```python
from build123d import *

# Parameters (mm, degrees)
SKETCH1_R           = 1.75
BOSS_EXTRUDE1_DEPTH = 12
SKETCH3_R           = 1.6
CUT_EXTRUDE1_DEPTH  = 3.5
BOSS_EXTRUDE2_DEPTH = 12


with BuildPart() as part:
    # Sketch1 → Boss-Extrude1 (new body)
    with BuildSketch(Plane(origin=(0, 0, 0), x_dir=(1, 0, 0), z_dir=(0, 1, 0))):
        Polygon((-1.649648438, 29.291322314), (-1.649648438, -3.708677686), (3.350351562, -3.708677686), (3.350351562, 31.791322314), (-26.649648438, 31.791322314), (-26.649648438, 29.291322314), align=None)
        with Locations((0.850351562, -1.208677686)):
            Circle(SKETCH1_R, mode=Mode.SUBTRACT)
    extrude(amount=BOSS_EXTRUDE1_DEPTH)

    # Sketch3 → Cut-Extrude1 (cut, through all)
    with BuildSketch(Plane.XY.offset(-29.291322314)):
        with Locations((-21.379789069, 2.5)):
            Circle(SKETCH3_R)
        with Locations((-21.379789069, 9.5)):
            Circle(SKETCH3_R)
    extrude(amount=-CUT_EXTRUDE1_DEPTH, mode=Mode.SUBTRACT)

    # Sketch4 → Boss-Extrude2 (add, through all)
    with BuildSketch(Plane(origin=(0, 0, 0), x_dir=(1, 0, 0), z_dir=(0, 1, 0))):
        Polygon((-1.649648438, 4.291322314), (-4.149648438, 4.291322314), (-4.149648438, -6.208677686), (5.850351562, -6.208677686), (5.850351562, 3.519074646), (3.350351562, 3.519074646), (3.350351562, -3.708677686), (-1.649648438, -3.708677686), align=None)
    extrude(amount=BOSS_EXTRUDE2_DEPTH)


solid = part.part
```
Design review of the part built by this model. Coordinates are the model's own, in mm. A direction names the side the tool comes from. Coordinates: 2 decimals unless noted, no trailing zeros. Order: outer loops, then holes, each group sorted by start corner. A loop starts at its lowest first (then second) coordinate and runs counter-clockwise, first axis right, second up.
1) Take a section at C-C, the plane z = -21.5. Give the boundary of the cut face in (x, y), and give its area (3 significant figures).
2) Take a section at A-A, the plane y = 2. Give the boundary of the cut face in (x, z), and give its area (3 significant figures).
3) Take a section at B-B, the plane y = 7. Give the boundary of the cut face in (x, z), and give its area (3 significant figures).
4) For faces 5 (the flat face through (-4.15, 6, 1)), 6 (the flat face through (5, 6, -3.519)), 7 (the flat face through (-3, 6, -4.291)), list the 3-axis set-ups (+Z, -Z, +X, -X, +Y, -Y) from which the entire face can be reached by the end or side of a thin tool; tool diameter is ignored.
5) Take a section at D-D, the plane x = -13. Give the boundary of the cut face in (y, z).
6) Mouldability with a two-part tool opening along Z and no side actions: class faces 1 (the flat face through (-1.65, 6, -17)), 2 (the flat face through (1, 6, 6.209)), 3 (the cylindrical face through (-0.54, 5.92, 2.27)), 4 (the flat face through (-1, 0, -16)) as +Z half, -Z half, draft (parallel to the pull), parting line (faces both ways), or undercut.
7) Wall thickness on line 1 along Z through (x, y) = (-3.5, 10.75); line 2 along Z through (x, y) = (-10, 4.75); line 3 along X through (y, z) = (0.5, -9): over which ranges is each line inside the solid? List them lowest first.
8) Clearance check with flat-ended pins moving along their axes: pin 1 (3.5 mm diameter, centred on x = -20, y = 3.5, fed in from +Z); pin 2 (3.5 mm diameter, centred on y = 3, z = -12, fed in from +X); pin 3 (0.8 mm diameter, centred on x = 5, y = 4, fed in from -Z); pin 4 (1.9 mm diameter, centred on x = -21.38, y = 9.5, fed in from -Z). State where each tip first meets the part, or that it passes through.
Returned:
1. outline: (-1.65, 0) - (3.35, 0) - (3.35, 12) - (-1.65, 12) - close
1. area: 60.0 mm2
2. outline: (-26.65, -31.79) - (-22.9, -31.79) - (-22.9, -29.29) - (-26.65, -29.29) - close; (-19.86, -31.79) - (3.35, -31.79) - (3.35, -3.52) - (5.85, -3.52) - (5.85, 6.21) - (-4.15, 6.21) - (-4.15, -4.29) - (-1.65, -4.29) - (-1.65, -29.29) - (-19.86, -29.29) - close; hole circle Ø3.5 at (0.85, 1.21)
2. area: 286 mm2
3. outline: (-26.65, -31.79) - (3.35, -31.79) - (3.35, -3.52) - (5.85, -3.52) - (5.85, 6.21) - (-4.15, 6.21) - (-4.15, -4.29) - (-1.65, -4.29) - (-1.65, -29.29) - (-26.65, -29.29) - close; hole circle Ø3.5 at (0.85, 1.21)
3. area: 293 mm2
4. face 5: +Z, -X, +Y, -Y
4. face 6: -Z, +X, +Y, -Y
4. face 7: -X, +Y, -Y
5. outline: (0, -31.79) - (12, -31.79) - (12, -29.29) - (0, -29.29) - close
6. face 1: undercut
6. face 2: +Z half
6. face 3: undercut
6. face 4: draft
7. line 1: z = -31.79 to -29.29, -4.29 to 6.21
7. line 2: z = -31.79 to -29.29
7. line 3: x = -1.65 to 3.35
8. pin 1: stops at z = -29.29
8. pin 2: stops at x = 3.35
8. pin 3: stops at z = -3.52
8. pin 4: passes through
